The drawing under review shows one solid part. Ordinate dimensions are in mm from its lowest x, y, z. Round coordinates to 2 decimals unless told otherwise and drop trailing zeros. Write each loop counter-clockwise with the first axis right and the second up, starting at its lowest first coordinate (ties: lowest second). Pieces come first, ordered by that corner, then holes. Notation, with made-up numbers: M 60.5,17 L 65.5,17 A18 ccw 65.5,42 Z; hole C -30.5,-9 d1. An arc over 180 degrees is marked long. One line per item, written item: value. Start each with the question number.
1) Mouldability with a two-part tool opening along X and no side actions: class the marked faces 1, 2, 3 and 4 as +X half, -X half, draft (parallel to the pull), parting line (faces both ways), or undercut.
2) Take a section at D-D, the plane y = 65. Write out the cut boundary in (x, z), and give its area (3 significant figures).
3) Take a section at A-A, the plane x = 40. Write out the cut boundary in (y, z).
4) Take a section at B-B, the plane z = 10. Write out the cut boundary in (x, y), and give its area (3 significant figures).
5) For P1, Ø2.5, axis at x = 11, z = 12, coming from the +Y side, flat-tipped, find the tip position at first contact; note if it passes through.
6) Wall thickness on probe 1 along Y at (x, z) = (40, 11.25); probe 2 along Z at (x, y) = (40, 76.5); probe 3 along Y at (x, z) = (30, 7.5): over which ranges is each line inside the solid? List them lowest first.
7) Take a section at C-C, the plane y = 40. Write out the cut boundary in (x, z), and give its area (3 significant figures).
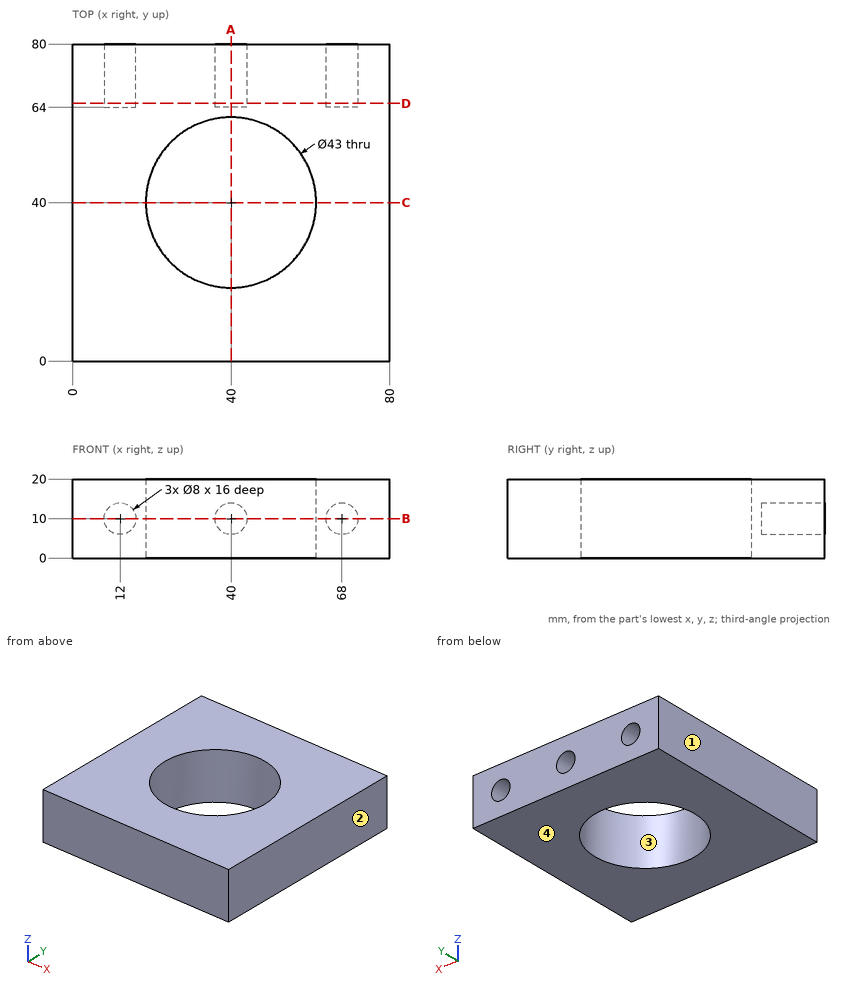
Checked values:
1. face 1: -X half
1. face 2: +X half
1. face 3: undercut
1. face 4: draft
2. outline: M 0,0 L 80,0 L 80,20 L 0,20 Z; hole C 12,10 d8; hole C 40,10 d8; hole C 68,10 d8
2. area: 1,450 mm2
3. outline: M 0,0 L 18.5,0 L 18.5,20 L 0,20 Z; M 61.5,0 L 80,0 L 80,6 L 64,6 L 64,14 L 80,14 L 80,20 L 61.5,20 Z
4. outline: M 0,0 L 80,0 L 80,80 L 72,80 L 72,64 L 64,64 L 64,80 L 44,80 L 44,64 L 36,64 L 36,80 L 16,80 L 16,64 L 8,64 L 8,80 L 0,80 Z; hole C 40,40 d43
4. area: 4,560 mm2
5. P1: stops at y = 64
6. probe 1: y = 0 to 18.5, 61.5 to 64
6. probe 2: z = 0 to 6, 14 to 20
6. probe 3: y = 0 to 20.97, 59.03 to 80
7. outline: M 0,0 L 18.5,0 L 18.5,20 L 0,20 Z; M 61.5,0 L 80,0 L 80,20 L 61.5,20 Z
7. area: 740 mm2
